Could you check a few things on this model? Use its own coordinates, in mm. A direction names the side the tool comes from. Round coordinates to 2 decimals unless told otherwise and drop trailing zeros. Loops run counter-clockwise (first coordinate to the right, second up) from the corner with the lowest first, then second, coordinate; pieces in that order, holes last. Notation, with made-up numbers: (-26, -23) -> (11, -23) arc R13 cw to (11, -12) -> close; hole circle Ø6 at (3.25, 24.25). An arc over 180 degrees is marked (long way). One line per item, written item: value.
```python
from build123d import *

# Parameters (mm, degrees)
SKETCH_1_W               = 34
SKETCH_1_H               = 20
EXTRUDE_1_DEPTH          = 22.7
SKETCH_2_R               = 8
EXTRUDE_2_DEPTH          = 3
SKETCH_3_R               = 1
CUT_EXTRUDE_1_DEPTH      = 6
CUT_EXTRUDE_START        = -6
SKETCH_5_R               = 1
CUT_EXTRUDE_2_DEPTH      = 6
SKETCH_6_R               = 5
CUT_EXTRUDE_3_DEPTH      = 1
SKETCH_7_R               = 2.5
CUT_EXTRUDE_4_DEPTH      = 2
SKETCH_8_W               = 10
SKETCH_8_H               = 9
CUT_EXTRUDE_5_DEPTH      = 3.8
SKETCH_9_R               = 1.25
CUT_EXTRUDE_6_DEPTH      = 3.8
SKETCH_10_R              = 1
CUT_EXTRUDE_7_DEPTH      = 6
PATTERN_CIRCULAR_1_COUNT = 4


with BuildPart() as part:
    # 草图1 → 凸台-拉伸1 (new body)
    with BuildSketch(Plane.XY):
        Rectangle(SKETCH_1_W, SKETCH_1_H)
    extrude(amount=EXTRUDE_1_DEPTH)

    # 草图2 → 凸台-拉伸2 (add)
    with BuildSketch(Plane.XY.offset(22.7)):
        with Locations(Location((7.5, 0, 0), (0, 0, 180))):
            Circle(SKETCH_2_R)
    extrude(amount=EXTRUDE_2_DEPTH)

    # 草图3 → 切除-拉伸1 (cut)
    with BuildSketch(Plane.XY.offset(22.7)):
        with Locations((-15, 8)):
            Circle(SKETCH_3_R)
        with Locations((15, 8)):
            Circle(SKETCH_3_R)
        with Locations((-15, -8)):
            Circle(SKETCH_3_R)
        with Locations((15, -8)):
            Circle(SKETCH_3_R)
    extrude(amount=-CUT_EXTRUDE_1_DEPTH, mode=Mode.SUBTRACT)

    # 草图5 → 切除-拉伸2 (cut)
    with BuildSketch(Plane(origin=(0, 0, 0), x_dir=(-1, 0, 0), z_dir=(0, 0, -1)).offset(CUT_EXTRUDE_START)):
        with Locations(Location((-15, 8, 0), (0, 0, 180))):
            Circle(SKETCH_5_R)
        with Locations(Location((15, 8, 0), (0, 0, 180))):
            Circle(SKETCH_5_R)
        with Locations(Location((-15, -8, 0), (0, 0, 180))):
            Circle(SKETCH_5_R)
        with Locations(Location((15, -8, 0), (0, 0, 180))):
            Circle(SKETCH_5_R)
    extrude(amount=CUT_EXTRUDE_2_DEPTH, mode=Mode.SUBTRACT)

    # 草图6 → 切除-拉伸3 (cut)
    with BuildSketch(Plane(origin=(0, 0, 0), x_dir=(-1, 0, 0), z_dir=(0, 0, -1))):
        with Locations((-7.5, 0)):
            Circle(SKETCH_6_R)
    extrude(amount=-CUT_EXTRUDE_3_DEPTH, mode=Mode.SUBTRACT)

    # 草图7 → 切除-拉伸4 (cut)
    with BuildSketch(Plane(origin=(0, 0, 1), x_dir=(-1, 0, 0), z_dir=(0, 0, -1))):
        with Locations((-7.5, 0)):
            Circle(SKETCH_7_R)
    extrude(amount=-CUT_EXTRUDE_4_DEPTH, mode=Mode.SUBTRACT)

    # 草图8 → 切除-拉伸5 (cut)
    with BuildSketch(Plane(origin=(0, 10, 0), x_dir=(1, 0, 0), z_dir=(0, 1, 0))):
        with Locations((-2, -4.5)):
            Rectangle(SKETCH_8_W, SKETCH_8_H)
    cut_extrude_5 = extrude(amount=-CUT_EXTRUDE_5_DEPTH, mode=Mode.SUBTRACT)

    # 镜向1: 切除-拉伸5 across plane
    add(cut_extrude_5.mirror(Plane.ZX), mode=Mode.SUBTRACT)

    # 草图9 → 切除-拉伸6 (cut)
    with BuildSketch(Plane(origin=(0, 0, 3), x_dir=(-1, 0, 0), z_dir=(0, 0, -1))):
        with Locations((-7.5, 0)):
            Circle(SKETCH_9_R)
    extrude(amount=-CUT_EXTRUDE_6_DEPTH, mode=Mode.SUBTRACT)

    # 草图10 → 切除-拉伸7 (cut)
    with BuildSketch(Plane.XY.offset(25.7)):
        with Locations((13.5, 0)):
            Circle(SKETCH_10_R)
    cut_extrude_7 = extrude(amount=-CUT_EXTRUDE_7_DEPTH, mode=Mode.SUBTRACT)

    # 阵列(圆周)1: 切除-拉伸7 ×4 about axis
    pattern_circular_1_axis = Axis((7.5, 0, 0), (0, 0, 1))
    for i in range(1, PATTERN_CIRCULAR_1_COUNT):
        add(cut_extrude_7.rotate(pattern_circular_1_axis, i * 360 / PATTERN_CIRCULAR_1_COUNT), mode=Mode.SUBTRACT)


solid = part.part
```
Item 1: If we section it at D-D on y = 0: List the corners of the cut face in (x, z) for me.
Output:
outline: (-17, 0) -> (2.5, 0) -> (2.5, 1) -> (5, 1) -> (5, 3) -> (6.25, 3) -> (6.25, 6.8) -> (8.75, 6.8) -> (8.75, 3) -> (10, 3) -> (10, 1) -> (12.5, 1) -> (12.5, 0) -> (17, 0) -> (17, 22.7) -> (15.5, 22.7) -> (15.5, 25.7) -> (14.5, 25.7) -> (14.5, 19.7) -> (12.5, 19.7) -> (12.5, 25.7) -> (2.5, 25.7) -> (2.5, 19.7) -> (0.5, 19.7) -> (0.5, 25.7) -> (-0.5, 25.7) -> (-0.5, 22.7) -> (-17, 22.7) -> close
Item 2: I need wall thicknesses on line 1 (Y direction, x = 15, z = 3.1); line 2 (X direction, y = -0.25, z = 19.75); line 3 (X direction, y = 7.25, z = 19.75). Which ranges of each line are inside material? Lowest first, please. Write a range as from..to.
Output:
line 1: y = -10..-9, -7..7, 9..10
line 2: x = -17..0.53, 2.47..12.53, 14.47..17
line 3: x = -17..-15.66, -14.34..14.34, 15.66..17
Item 3: If we mould it in two halves opening along X, with no side actions, what happens to faces 1 (the face through (0, -10, 11)), 2 (the face through (8.75, 0.05, 4.87)), 3 (the face through (17, 0, 11))? For each: released by +X, released by -X, zero draft, split by the parting line, or undercut.
Output:
face 1: zero draft
face 2: undercut
face 3: released by +X
Item 4: If we section it at B-B on x = 7.5: List the corners of the cut face in (y, z) for me, plus the area to 4 significant figures.
Output:
outline: (-10, 0) -> (-5, 0) -> (-5, 1) -> (-2.5, 1) -> (-2.5, 3) -> (-1.25, 3) -> (-1.25, 6.8) -> (1.25, 6.8) -> (1.25, 3) -> (2.5, 3) -> (2.5, 1) -> (5, 1) -> (5, 0) -> (10, 0) -> (10, 22.7) -> (8, 22.7) -> (8, 25.7) -> (7, 25.7) -> (7, 19.7) -> (5, 19.7) -> (5, 25.7) -> (-5, 25.7) -> (-5, 19.7) -> (-7, 19.7) -> (-7, 25.7) -> (-8, 25.7) -> (-8, 22.7) -> (-10, 22.7) -> close
area: 448.5 mm²
Item 5: If we section it at A-A on z = 7.5: List the corners of the cut face in (x, y) for me, plus the area to 3 significant figures.
Output:
outline: (-17, -10) -> (-7, -10) -> (-7, -6.2) -> (3, -6.2) -> (3, -10) -> (17, -10) -> (17, 10) -> (3, 10) -> (3, 6.2) -> (-7, 6.2) -> (-7, 10) -> (-17, 10) -> close
area: 604 mm²
Item 6: For faces 4 (the face through (-2, 6.2, 4)), 5 (the face through (15, 8, 6)), 6 (the face through (13, 0, 19.7)), which set-ups out of +Z, -Z, +X, -X, +Y, -Y let a thin tool reach every point of the face, with its end or its side?
Output:
face 4: -Z, +Y
face 5: -Z
face 6: +Z
Item 7: Will these pins go through, and if not, where does the flat tip stop? pin 1 Ø5.5 at (x, y) = (8, 1) entering from -Z; pin 2 Ø1.6 at (x, y) = (7.5, 6) entering from +Z; pin 3 Ø2 at (x, y) = (-5, -3) entering from +Z.
Output:
pin 1: stops at z = 1
pin 2: stops at z = 19.7
pin 3: stops at z = 22.7
Item 8: If we section it at C-C on z = 2.25: List the corners of the cut face in (x, y) for me.
Output:
outline: (-17, -10) -> (-7, -10) -> (-7, -6.2) -> (3, -6.2) -> (3, -10) -> (17, -10) -> (17, 10) -> (3, 10) -> (3, 6.2) -> (-7, 6.2) -> (-7, 10) -> (-17, 10) -> close; hole circle Ø2 at (-15, -8); hole circle Ø2 at (-15, 8); hole circle Ø5 at (7.5, 0); hole circle Ø2 at (15, -8); hole circle Ø2 at (15, 8)
